The listing builds one solid part. Answer for the finished solid, in the listing's coordinates (mm). Face numbers are marked on the shaded views. Coordinates: 2 decimals unless noted, no trailing zeros. Order: outer loops, then holes, each group sorted by start corner. A loop starts at its lowest first (then second) coordinate and runs counter-clockwise, first axis right, second up.
from build123d import *

# Parameters (mm, degrees)
SKETCH_2_R      = 1.5
EXTRUDE_1_DEPTH = 3


with BuildPart() as part:
    # 草圖2 → 填料-伸長1 (new body)
    with BuildSketch(Plane.XY):
        with BuildLine():
            Line((2198.740145456, 1572.08621907), (2198.740145456, 1577.10008841))
            ThreePointArc((2198.740145456, 1577.10008841), (2194.740145456, 1581.10008841), (2190.740145456, 1577.10008841))
            Line((2190.740145456, 1577.10008841), (2190.740145457, 1572.15435767))
            Line((2190.740145457, 1572.15435767), (2190.740145457, 1571.15435767))
            Line((2190.740145457, 1571.15435767), (2190.740145456, 1541.250580548))
            Line((2190.740145456, 1541.250580548), (2190.740145456, 1540.250580548))
            Line((2190.740145456, 1540.250580548), (2190.740145456, 1516.623912375))
            Line((2190.740145456, 1516.623912375), (2190.740145456, 1515.623912375))
            Line((2190.740145456, 1515.623912375), (2190.740145455, 1497.10018841))
            ThreePointArc((2190.740145455, 1497.10018841), (2194.740095455, 1493.100088408), (2198.740145455, 1497.100088412))
            Line((2198.740145455, 1497.100088412), (2198.740145456, 1515.966387039))
            Line((2198.740145456, 1515.966387039), (2198.740145456, 1516.966387039))
            Line((2198.740145456, 1516.966387039), (2198.740145456, 1541.60008841))
            Line((2198.740145456, 1541.60008841), (2198.740145456, 1542.60008841))
            Line((2198.740145456, 1542.60008841), (2198.740145456, 1571.08621907))
            Line((2198.740145456, 1571.08621907), (2198.740145456, 1572.08621907))
        make_face()
        with Locations((2194.740145455, 1497.100088409)):
            Circle(SKETCH_2_R, mode=Mode.SUBTRACT)
        with Locations((2194.740195453, 1577.100138407)):
            Circle(SKETCH_2_R, mode=Mode.SUBTRACT)
    extrude(amount=EXTRUDE_1_DEPTH)


solid = part.part
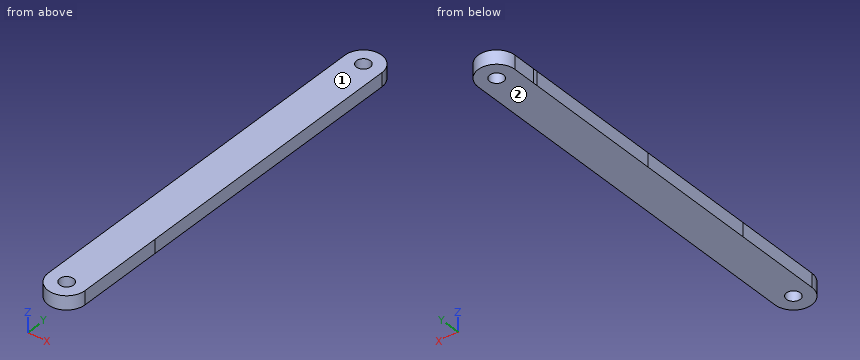
(1) Find section B-B on x = 2197. Determine the outline of the cut face in (y, z).
(2) Given pin 1 Ø2.5 at (x, y) = (2194.74, 1577.1) entering from -Z, flat-ended and moving along its own axis, determine where the tip first touches the part or whether it passes through.
(3) Find the intervals of material crossed by probe 1 along Y at (x, z) = (2193.75, 0.75); probe 2 along Y at (x, z) = (2194.5, 0.7); probe 3 along Y at (x, z) = (2197.25, 0.35), in increasing order.
(4) The mould has two halves that part along Z. Classify the marked faces 1 and 2: pulls with the +Z half, pulls with the -Z half, needs draft (parallel to the pull), parting line crosses it, or undercut.
(5) Find section A-A on z = 2.45. Determine the outline of the cut face in (x, y).
(6) Find section C-C on x = 2192.25. Determine the outline of the cut face in (y, z), then the cut area to 3 significant figures.
Resolved:
1. outline: (1493.8, 0) - (1580.4, 0) - (1580.4, 3) - (1493.8, 3) - close
2. pin 1: passes through
3. probe 1: y = 1493.22 to 1495.97, 1498.23 to 1575.97, 1578.23 to 1580.98
3. probe 2: y = 1493.11 to 1495.62, 1498.58 to 1575.62, 1578.58 to 1581.09
3. probe 3: y = 1493.99 to 1580.21
4. face 1: pulls with the +Z half
4. face 2: pulls with the -Z half
5. outline: (2190.74, 1497.1) arc R4 ccw to (2198.74, 1497.1) - (2198.74, 1577.1) arc R4 ccw to (2190.74, 1577.1) - close; hole circle Ø3 at (2194.74, 1497.1); hole circle Ø3 at (2194.74, 1577.1)
6. outline: (1493.97, 0) - (1580.23, 0) - (1580.23, 3) - (1493.97, 3) - close
6. area: 259 mm2
